The listing builds one solid part. Answer for the finished solid, in the listing's coordinates (mm). A direction names the side the tool comes from. Coordinates: 2 decimals unless noted, no trailing zeros.
from build123d import *

# Parameters (mm, degrees)
SKETCH1_R           = 15
BOSS_EXTRUDE1_DEPTH = 17
CIRPATTERN1_COUNT   = 4
BOSS_EXTRUDE3_DEPTH = 10
SKETCH12_W          = 14.047466192
SKETCH12_H          = 9.954867113
CUT_EXTRUDE2_DEPTH  = 3
CUT_EXTRUDE3_DEPTH  = 9
CIRPATTERN11_COUNT  = 4
SKETCH14_R          = 12.072799678
CUT_EXTRUDE4_DEPTH  = 24


with BuildPart() as part:
    # Sketch1 → Boss-Extrude1 (new body)
    with BuildSketch(Plane(origin=(0, 0, 0), x_dir=(1, 0, 0), z_dir=(0, 1, 0))):
        Circle(SKETCH1_R)
    extrude(amount=BOSS_EXTRUDE1_DEPTH)

    # Sketch7 → Loft3 section 0
    with BuildSketch(Plane(origin=(0, 17, 0), x_dir=(1, 0, 0), z_dir=(0, 1, 0))):
        with BuildLine():
            Line((-15.419212864, -8.429185203), (-13.785295759, -5.913173499))
            Line((-13.785295759, -5.913173499), (-0.036662397, -14.999955196))
            Line((-0.036662397, -14.999955196), (-1.670579502, -17.515966899))
            ThreePointArc((-1.670579502, -17.515966899), (-5.449846484, -15.759052669), (-8.767392344, -13.236455593))
            ThreePointArc((-8.767392344, -13.236455593), (-12.350066375, -11.188104454), (-15.419212864, -8.429185203))
        make_face()
    # Sketch2 → Loft3 section 1
    with BuildSketch(Plane.XZ):
        with BuildLine():
            Line((8.1969132, 15.523322087), (8.1969132, 12.562269461))
            Line((8.1969132, 12.562269461), (-8.1969132, 12.562269461))
            Line((-8.1969132, 12.562269461), (-8.1969132, 15.562269461))
            ThreePointArc((-8.1969132, 15.562269461), (-4.120295252, 16.204516854), (0, 15.971144539))
            ThreePointArc((0, 15.971144539), (4.122381552, 16.185154095), (8.1969132, 15.523322087))
        make_face()
    loft3 = loft()

    # CirPattern1: Loft3 ×4 about axis
    cirpattern1_axis = Axis((0, 0, 0), (0, -1, 0))
    for i in range(1, CIRPATTERN1_COUNT):
        add(loft3.rotate(cirpattern1_axis, i * 360 / CIRPATTERN1_COUNT))

    # Sketch8 → Boss-Extrude3 (add)
    with BuildSketch(Plane(origin=(0, 17, 0), x_dir=(1, 0, 0), z_dir=(0, 1, 0))):
        with BuildLine():
            Line((17.572799678, 0), (12.072799678, 0))
            ThreePointArc((12.072799678, 0), (8.536758521, -8.536758521), (0, -12.072799678))
            Line((0, -12.072799678), (0, -17.572799678))
            ThreePointArc((0, -17.572799678), (12.425845817, -12.425845817), (17.572799678, 0))
        make_face()
    boss_extrude3 = extrude(amount=BOSS_EXTRUDE3_DEPTH)

    # Sketch12 → Cut-Extrude2 (cut)
    with BuildSketch(Plane.ZY):
        with Locations((15, 26.710348928)):
            Rectangle(SKETCH12_W, SKETCH12_H)
    cut_extrude2 = extrude(amount=-CUT_EXTRUDE2_DEPTH, mode=Mode.SUBTRACT)

    # Sketch13 → Cut-Extrude3 (cut)
    with BuildSketch(Plane(origin=(7.536399839, 0, 5.847061058), x_dir=(-0.612987567, 0, 0.790092553), z_dir=(-0.790092553, 0, -0.612987567))):
        Polygon((-4.655510065, 27), (7.400476101, 21.732915371), (11.841354417, 21.732915371), (11.841354417, 27), align=None)
    cut_extrude3 = extrude(amount=-CUT_EXTRUDE3_DEPTH, mode=Mode.SUBTRACT)

    # CirPattern11: Boss-Extrude3, Cut-Extrude2, Cut-Extrude3 ×4 about axis
    cirpattern11_axis = Axis((0, 0, 0), (0, 1, 0))
    for i in range(1, CIRPATTERN11_COUNT):
        add(boss_extrude3.rotate(cirpattern11_axis, i * 360 / CIRPATTERN11_COUNT))
        add(cut_extrude2.rotate(cirpattern11_axis, i * 360 / CIRPATTERN11_COUNT), mode=Mode.SUBTRACT)
        add(cut_extrude3.rotate(cirpattern11_axis, i * 360 / CIRPATTERN11_COUNT), mode=Mode.SUBTRACT)

    # Sketch14 → Cut-Extrude4 (cut)
    with BuildSketch(Plane(origin=(0, 17, 0), x_dir=(1, 0, 0), z_dir=(0, 1, 0))):
        Circle(SKETCH14_R)
    extrude(amount=-CUT_EXTRUDE4_DEPTH, mode=Mode.SUBTRACT)


solid = part.part
1) Determine the mould class of faces 4 (the face through (-3, 21.733, -15)), 5 (the face through (9.84, 24.403, -10.582)), 6 (the face through (15, 24, 0)) for opening direction X: released by +X, released by -X, zero draft, split by the parting line, or undercut.
2) Consider L1, parallel to X at y = 4, z = 0; L2, parallel to Z at x = -8, y = 20; L3, parallel to X at y = 6.5, z = 4. Determine where each line is inside the solid, lowest interval first.
3) A tool of negligible diameter and unlimited length cuts with its end or side. For faces 1 (the face through (13.25, 8.38, -7.03)), 2 (the face through (-9, 17, 14)), 3 (the face through (9, 17, -14)), from which of +Z, -Z, +X, -X, +Y, -Y can it reach the whole face along a straight path? Write none if from no direction.
4) Each of these flat-tipped pins is pushed along its axis until it touches: P1, Ø4, axis at x = 12, z = -13.5, coming from the +Y side; P2, Ø6, axis at y = 9.5, z = 8.5, coming from the -X side; P3, Ø4, axis at y = 24.5, z = -15, coming from the -X side; P4, Ø19.5, axis at x = 0, z = 0, coming from the -Y side. Where does it stop, or does it pass through?
Filled sheet:
1. face 4: undercut
1. face 5: released by +X
1. face 6: zero draft
2. L1: x = -15.83 to -12.07, 12.07 to 15.83
2. L2: z = -15.65 to -9.04, 9.04 to 15.65
2. L3: x = -16.3 to -11.39, 11.39 to 14.88
3. face 1: +X
3. face 2: +Z, -X
3. face 3: -Z, +X
4. P1: stops at y = 25.29
4. P2: stops at x = -13.96
4. P3: stops at x = -11.49
4. P4: passes through
